For this review, take the finished solid that the model builds, in its own axes (mm). A direction names the side the tool comes from. Give positions to 0.01 mm unless a question says otherwise; leave off trailing zeros. Write each loop counter-clockwise with the first axis right and the second up, starting at its lowest first coordinate (ties: lowest second). Pieces come first, ordered by that corner, then holes.
1) For P1, Ø1.6, axis at x = 36, y = 9, coming from the +Z side, flat-tipped, find the tip position at first contact; note if it passes through.
2) We need section B-B on z = 3.1. Give the boundary of the cut face in (x, y).
3) Machinability: for faces 4 (the face through (10.186, 9.361, 3.014)), 5 (the face through (14.169, 8.526, 0.986)), which of the approach directions +Z, -Z, +X, -X, +Y, -Y give a long, thin tool a straight path to every point of the face, cutting with its end or side? Answer none if there is none.
4) We need section C-C on y = 7.25. Give the boundary of the cut face in (x, z).
5) Wall thickness on line 1 along Y through (x, z) = (12.5, 0.65); line 2 along X through (y, z) = (8, 1.3); line 3 along Y through (x, z) = (37.5, 2.5): over which ranges is each line inside the solid? List them lowest first.
6) We need section A-A on x = 37.5. Give the boundary of the cut face in (y, z), and give its area (3 significant figures).
7) Draft analysis for pull direction X (two halves, no side actions). For faces 1 (the face through (35.16, 6.68, 3.01)), 2 (the face through (25, 0, 2)), 3 (the face through (50, 7, 2)), state which applies: pulls with the +X half, pulls with the -X half, needs draft (parallel to the pull), parting line crosses it, or undercut.
from build123d import *

# Parameters (mm, degrees)
SKETCH1_W                 = 50
SKETCH1_H                 = 14
SKETCH1_R                 = 1.75
BOSS_EXTRUDE1_DEPTH       = 4
NUTHOLECUT_EXTRUDE1_DEPTH = 2


with BuildPart() as part:
    # Sketch1 → Boss-Extrude1 (new body)
    with BuildSketch(Plane.XY):
        with Locations((25, 7)):
            Rectangle(SKETCH1_W, SKETCH1_H)
        with Locations((12.5, 8)):
            Circle(SKETCH1_R, mode=Mode.SUBTRACT)
        with Locations((37.5, 8)):
            Circle(SKETCH1_R, mode=Mode.SUBTRACT)
    extrude(amount=BOSS_EXTRUDE1_DEPTH)

    # NutHoleSketch7 → NutHoleCut-Extrude1 (cut)
    with BuildSketch(Plane.XY.offset(4)):
        Polygon((14.05, 5.315321248), (15.6, 8), (14.05, 10.684678752), (10.95, 10.684678752), (9.4, 8), (10.95, 5.315321248), align=None)
        Polygon((39.05, 5.315321248), (40.6, 8), (39.05, 10.684678752), (35.95, 10.684678752), (34.4, 8), (35.95, 5.315321248), align=None)
    extrude(amount=-NUTHOLECUT_EXTRUDE1_DEPTH, mode=Mode.SUBTRACT)


solid = part.part
Results list:
1. P1: stops at z = 2
2. outline: (0, 0) - (50, 0) - (50, 14) - (0, 14) - close; hole (9.4, 8) - (10.95, 5.32) - (14.05, 5.32) - (15.6, 8) - (14.05, 10.68) - (10.95, 10.68) - close; hole (34.4, 8) - (35.95, 5.32) - (39.05, 5.32) - (40.6, 8) - (39.05, 10.68) - (35.95, 10.68) - close
3. face 4: +Z
3. face 5: +Z, -Z
4. outline: (0, 0) - (10.92, 0) - (10.92, 2) - (9.83, 2) - (9.83, 4) - (0, 4) - close; (14.08, 0) - (35.92, 0) - (35.92, 2) - (34.83, 2) - (34.83, 4) - (15.17, 4) - (15.17, 2) - (14.08, 2) - close; (39.08, 0) - (50, 0) - (50, 4) - (40.17, 4) - (40.17, 2) - (39.08, 2) - close
5. line 1: y = 0 to 6.25, 9.75 to 14
5. line 2: x = 0 to 10.75, 14.25 to 35.75, 39.25 to 50
5. line 3: y = 0 to 5.32, 10.68 to 14
6. outline: (0, 0) - (6.25, 0) - (6.25, 2) - (5.32, 2) - (5.32, 4) - (0, 4) - close; (9.75, 0) - (14, 0) - (14, 4) - (10.68, 4) - (10.68, 2) - (9.75, 2) - close
6. area: 38.3 mm2
7. face 1: undercut
7. face 2: needs draft
7. face 3: pulls with the +X half
